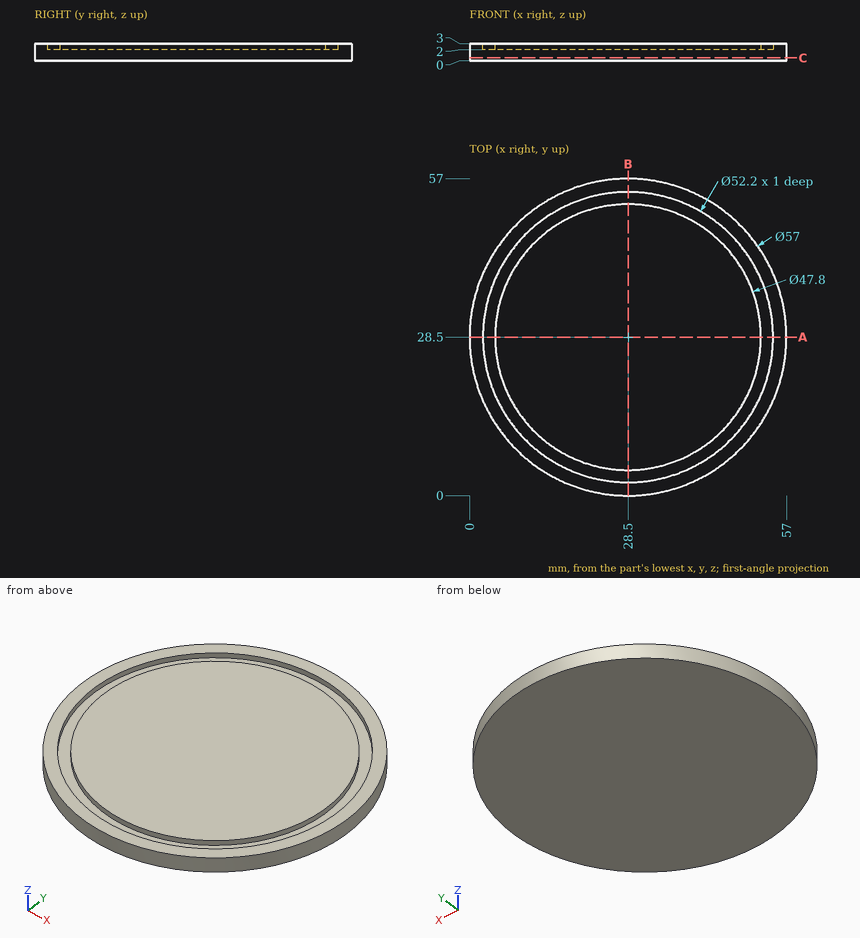
Geometry check sheet. Reference: drawing and pictorial views, mm from the part's lowest x, y, z. Coordinates: 2 decimals unless noted, no trailing zeros. Order: outer loops, then holes, each group sorted by start corner. A loop starts at its lowest first (then second) coordinate and runs counter-clockwise, first axis right, second up. Notation, with made-up numbers: (53, -36.75) -> (61, -36.75) arc R26 ccw to (61, -15.75) -> close; hole circle Ø8 at (-26.75, -26). An arc over 180 degrees is marked (long way). Write item = value, one per line. Start each with the question number.
1) Material ranges on L1, parallel to Y at x = 28.5, z = 2.6; L2, parallel to X at y = 19.5, z = 2.4; L3, parallel to X at y = 33, z = 2.6, recorded low to high.
2) Cross-section at A-A (y = 28.5). Enter the section's corners in (x, z).
3) Cross-section at C-C (z = 0.5). Enter the section's corners in (x, y), then the cut area to 3 significant figures.
Ans:
q1.L1 = 0 to 2.4, 4.6 to 52.4, 54.6 to 57
q1.L2 = 1.46 to 4, 6.36 to 50.64, 53 to 55.54
q1.L3 = 0.36 to 2.79, 5.03 to 51.97, 54.21 to 56.64
q2.outline = (0, 0) -> (57, 0) -> (57, 3) -> (54.6, 3) -> (54.6, 2) -> (52.4, 2) -> (52.4, 3) -> (4.6, 3) -> (4.6, 2) -> (2.4, 2) -> (2.4, 3) -> (0, 3) -> close
q3.outline = circle Ø57 at (28.5, 28.5)
q3.area = 2,550 mm²
